```python
from build123d import *

# Parameters (mm, degrees)
SKETCH1_R           = 1.778
SKETCH1_R_2         = 1.55
SKETCH1_R_3         = 6.35
BOSS_EXTRUDE1_DEPTH = 6.35
FILLET2_R           = 2
FILLET4_R           = 8


with BuildPart() as part:
    # Sketch1 → Boss-Extrude1 (new body)
    with BuildSketch(Plane.XY):
        with BuildLine():
            Line((47.626117997, 29.779), (-12, 29.779))
            Line((-12, 29.779), (-12, 14.779))
            Line((-12, 14.779), (-15.488554272, 8.145838605))
            ThreePointArc((-15.488554272, 8.145838605), (-11.243708258, -13.410034474), (10.72211713, -13.830625591))
            Line((10.72211713, -13.830625591), (47.626117997, 14.779))
            Line((47.626117997, 14.779), (47.626117997, 29.779))
        make_face()
        with Locations((-9.779, 0)):
            Circle(SKETCH1_R, mode=Mode.SUBTRACT)
        with Locations((0, -9.779)):
            Circle(SKETCH1_R, mode=Mode.SUBTRACT)
        with Locations((0, 9.779)):
            Circle(SKETCH1_R, mode=Mode.SUBTRACT)
        with Locations((9.779, 0)):
            Circle(SKETCH1_R, mode=Mode.SUBTRACT)
        with Locations((-2.373882003, 22.279)):
            Circle(SKETCH1_R_2, mode=Mode.SUBTRACT)
        with Locations((12.626117997, 22.279)):
            Circle(SKETCH1_R_2, mode=Mode.SUBTRACT)
        with Locations((27.626117997, 22.279)):
            Circle(SKETCH1_R_2, mode=Mode.SUBTRACT)
        with Locations((42.626117997, 22.279)):
            Circle(SKETCH1_R_2, mode=Mode.SUBTRACT)
        Circle(SKETCH1_R_3, mode=Mode.SUBTRACT)
    extrude(amount=BOSS_EXTRUDE1_DEPTH)

    # Fillet2
    fillet2_edges = [part.edges().sort_by_distance(p)[0] for p in [
        (47.626117997, 29.779, 3.175),
        (47.626117997, 14.779, 3.175),
    ]]
    fillet(fillet2_edges, radius=FILLET2_R)

    # Fillet4
    fillet4_edges = [part.edges().sort_by_distance(p)[0] for p in [
        (-12, 14.779, 3.175),
        (-12, 29.779, 3.175),
    ]]
    fillet(fillet4_edges, radius=FILLET4_R)


solid = part.part
```
Check sheet for the modelled part. Datum: model origin and axes. Units: mm. Round coordinates to 2 decimals unless told otherwise and drop trailing zeros. Order: outer loops, then holes, each group sorted by start corner. A loop starts at its lowest first (then second) coordinate and runs counter-clockwise, first axis right, second up. Notation, with made-up numbers: (89.5, -14.5) -> (141.5, -14.5) arc R30 ccw to (141.5, 18.5) -> close; hole circle Ø10 at (62.25, 81). An arc over 180 degrees is marked (long way). One line per item, written item: value. Start each with the question number.
Q1. Cross-section at B-B (z = 1.75). Give the number of separate pieces and of enclosed holes in the cut face, and give its area (3 significant figures).
Q2. Cross-section at D-D (x = 13.5). Record the boundary of the cut face in (y, z).
Q3. Mould release check, pull along Y, two halves, no side actions. Record for faces 1 (the face through (47.025, 29.209, 3.219)), 2 (the face through (15, 12, 0)), 3 (the face through (-1.38, -6.2, 3.13)): pulls with the +Y half, pulls with the -Y half, needs draft (parallel to the pull), parting line crosses it, or undercut.
Q4. Cross-section at C-C (y = -4.5). Record the boundary of the cut face in (x, z).
Q5. Cross-section at A-A (x = 0). Record the boundary of the cut face in (y, z), and give its area (3 significant figures).
Q6. Thickness scan on line 1 (Y direction, x = 0, z = 1.5); line 2 (X direction, y = 0.5, z = 4); line 3 (X direction, y = 10, z = 3.5). Record the ranges inside material, lowest first.
Q7. Gauge pin test, flat ends, axial feed: pin 1 Ø2 at (x, z) = (9.5, 4) entering from -Y; pin 2 Ø2.5 at (y, z) = (18, 3.5) entering from -X. Record the tip position at first contact, or that the pin passes through.
Completed:
1. separate pieces: 1
1. enclosed holes: 9
1. area: 2,010 mm²
2. outline: (-11.68, 0) -> (21, 0) -> (21, 6.35) -> (-11.68, 6.35) -> close; (23.56, 0) -> (29.78, 0) -> (29.78, 6.35) -> (23.56, 6.35) -> close
3. face 1: pulls with the +Y half
3. face 2: needs draft
3. face 3: undercut
4. outline: (-16.91, 0) -> (-4.48, 0) -> (-4.48, 6.35) -> (-16.91, 6.35) -> close; (4.48, 0) -> (22.76, 0) -> (22.76, 6.35) -> (4.48, 6.35) -> close
5. outline: (-17.5, 0) -> (-11.56, 0) -> (-11.56, 6.35) -> (-17.5, 6.35) -> close; (-8, 0) -> (-6.35, 0) -> (-6.35, 6.35) -> (-8, 6.35) -> close; (6.35, 0) -> (8, 0) -> (8, 6.35) -> (6.35, 6.35) -> close; (11.56, 0) -> (29.78, 0) -> (29.78, 6.35) -> (11.56, 6.35) -> close
5. area: 174 mm²
6. line 1: y = -17.5 to -11.56, -8 to -6.35, 6.35 to 8, 11.56 to 29.78
6. line 2: x = -17.49 to -11.49, -8.07 to -6.33, 6.33 to 8.07, 11.49 to 29.21
6. line 3: x = -14.51 to -1.76, 1.76 to 41.46
7. pin 1: stops at y = -15.3
7. pin 2: stops at x = -12
